from build123d import *

# Parameters (mm, degrees)
F_8_0MM_DOWEL_HOLE1_D     = 8
F_8_0MM_DOWEL_HOLE1_DEPTH = 30
F_8_0MM_DOWEL_HOLE1_TIP   = 2.403442476
SKETCH10_R                = 2.75
CUT_EXTRUDE1_DEPTH        = 260
SKETCH11_R                = 2.75
CUT_EXTRUDE2_DEPTH        = 260
SKETCH12_R                = 4
CUT_EXTRUDE3_DEPTH        = 30


with BuildPart() as part:
    # Sketch1 → Revolve1 (revolve)
    with BuildSketch(Plane(origin=(0, 50, 0), x_dir=(1, 0, 0), z_dir=(0, 1, 0))):
        Polygon((85, -8), (0, -8), (0, -215), (8, -215), (8, -60), (6.5, -60), (6.5, -58), (8, -58), (8, -23), (85, -23), align=None)
    revolve(axis=Axis((0, 50, 8), (0, 0, 1)))

    # Ø8.0mm Dowel Hole1
    with Locations(Plane(origin=(0, 0, 8), x_dir=(-1, 0, 0), z_dir=(0, 0, -1))):
        with Locations((0, 95), (-38.97114317, 72.5), (-38.97114317, 27.5), (0, 5), (38.97114317, 27.5), (38.97114317, 72.5)):
            Hole(F_8_0MM_DOWEL_HOLE1_D / 2, depth=F_8_0MM_DOWEL_HOLE1_DEPTH)
            with Locations((0, 0, -(F_8_0MM_DOWEL_HOLE1_DEPTH + F_8_0MM_DOWEL_HOLE1_TIP / 2))):  # 118° drill point
                Cone(0, F_8_0MM_DOWEL_HOLE1_D / 2, F_8_0MM_DOWEL_HOLE1_TIP, mode=Mode.SUBTRACT)

    # Sketch10 → Cut-Extrude1 (cut)
    with BuildSketch(Plane(origin=(138.275547742, -79.833424711, 0), x_dir=(-0.5, -0.866025404, 0), z_dir=(0.866025404, -0.5, 0))):
        with Locations((-43.301270189, -125)):
            Circle(SKETCH10_R)
    extrude(amount=-CUT_EXTRUDE1_DEPTH, mode=Mode.SUBTRACT)

    # Sketch11 → Cut-Extrude2 (cut)
    with BuildSketch(Plane(origin=(46.091849247, 79.833424711, 0), x_dir=(0.866025404, -0.5, 0), z_dir=(0.5, 0.866025404, 0))):
        with Locations((-25, -125)):
            Circle(SKETCH11_R)
    extrude(amount=-CUT_EXTRUDE2_DEPTH, mode=Mode.SUBTRACT)

    # Sketch12 → Cut-Extrude3 (cut)
    with BuildSketch(Plane(origin=(0, 0, 8), x_dir=(-1, 0, 0), z_dir=(0, 0, -1))):
        with Locations((0, 50)):
            Circle(SKETCH12_R)
    extrude(amount=-CUT_EXTRUDE3_DEPTH, mode=Mode.SUBTRACT)


solid = part.part
Read the model definition and answer for the solid it produces. Units are mm, in the model's axes. A direction names the side the tool comes from. Give positions to 0.01 mm unless a question says otherwise; leave off trailing zeros. Loops run counter-clockwise (first coordinate to the right, second up) from the corner with the lowest first, then second, coordinate; pieces in that order, holes last. Notation, with made-up numbers: M 19,43 L 24,43 A24 cw 24,73 Z; hole C 42,64 d7. An arc over 180 degrees is marked long. Write each question's results on one line, items separated by ' | '.
1. Straight lines are drawn through the part: line 1 (Y direction, x = 0, z = 16.25); line 2 (Y direction, x = 0, z = 23.5); line 3 (Z direction, x = -24, y = 92). For each, find the intervals that lie inside material, in ascending order. Write a range as [from, to].
Values:
line 1: y = [-35, 1], [9, 46], [54, 91], [99, 135] | line 2: y = [42, 46], [54, 58] | line 3: z = [8, 23]
2. A tool of negligible diameter and unlimited length cuts with its end or side. For faces 1 (the face through (0.867, 46.095, 22.79)), 2 (the face through (-1.041, 57.932, 136.415)), 3 (the face through (-1.409, 43.655, 58.986)), from which of +Z, -Z, +X, -X, +Y, -Y can it reach the whole face along a straight path? Write none if from no direction.
Values:
face 1: -Z | face 2: +Z | face 3: none
3. The mould has two halves that part along Y. Classify faces 4 (the face through (-1, 32, 8)), 5 (the face through (-1.041, 57.932, 40.255)), 6 (the face through (0, 50, 38)): pulls with the +Y half, pulls with the -Y half, needs draft (parallel to the pull), parting line crosses it, or undercut.
Values:
face 4: needs draft | face 5: parting line crosses it | face 6: undercut
4. Given pin 1 (4 mm diameter, centred on x = 0, y = 51.5, fed in from -Z); pin 2 (1.5 mm diameter, centred on x = -33, y = 69.5, fed in from +Z); pin 3 (6 mm diameter, centred on y = 54.5, z = 175.5, fed in from -X), each flat-ended and moving along its own axis, determine where each tip first touches the part or whether it passes through.
Values:
pin 1: stops at z = 38 | pin 2: stops at z = 23 | pin 3: stops at x = -7.86
5. Section B-B on y = 5 is taken. Give the vertices of the cut face in (x, z), plus the area to 3 significant figures.
Values:
outline: M -72.11,8 L -4,8 L -4,23 L -72.11,23 Z; M 4,8 L 72.11,8 L 72.11,23 L 4,23 Z | area: 2,040 mm^2
6. Section D-D on y = -13.5 is taken. Give the vertices of the cut face in (x, z), plus the area to 3 significant figures.
Values:
outline: M -56.5,8 L 56.5,8 L 56.5,23 L -56.5,23 Z | area: 1,700 mm^2
7. Section C-C on z = 95.5 is taken. Give the vertices of the cut face in (x, y).
Values:
outline: C 0,50 d16
8. Section A-A on y = 27.5 is taken. Give the vertices of the cut face in (x, z), plus the area to 3 significant figures.
Values:
outline: M -81.97,8 L -42.97,8 L -42.97,23 L -81.97,23 Z; M -34.97,8 L 34.97,8 L 34.97,23 L -34.97,23 Z; M 42.97,8 L 81.97,8 L 81.97,23 L 42.97,23 Z | area: 2,220 mm^2
